Check sheet for the modelled part. Datum: model origin and axes. Units: mm. A direction names the side the tool comes from. Coordinates: 2 decimals unless noted, no trailing zeros. Loops run counter-clockwise (first coordinate to the right, second up) from the corner with the lowest first, then second, coordinate; pieces in that order, holes last. Notation, with made-up numbers: (-20, -24.75) -> (19, -24.75) arc R32 cw to (19, 7.25) -> close; hole circle Ø1 at (31, 58.25). An arc over 180 degrees is marked (long way). Use CSV: the item, a comma, the result in double quotes.
```python
from build123d import *

# Parameters (mm, degrees)
MODEL_R             = 2.5
MODEL_R_2           = 1.75
MODEL_W             = 40
MODEL_H             = 24
BOSS_EXTRUDE1_DEPTH = 12


with BuildPart() as part:
    # Model → Boss-Extrude1 (new body)
    with BuildSketch(Plane.XY):
        Polygon((5, 275), (0, 270), (0, 5), (5, 0), (125, 0), (130, 5), (130, 270), (125, 275), align=None)
        with Locations((16.49, 6.5)):
            Circle(MODEL_R, mode=Mode.SUBTRACT)
        with Locations((48.83, 6.5)):
            Circle(MODEL_R, mode=Mode.SUBTRACT)
        with Locations((81.17, 6.5)):
            Circle(MODEL_R, mode=Mode.SUBTRACT)
        with Locations((113.51, 6.5)):
            Circle(MODEL_R, mode=Mode.SUBTRACT)
        with Locations((29, 128.5)):
            Circle(MODEL_R_2, mode=Mode.SUBTRACT)
        with Locations((65, 128.5)):
            Circle(MODEL_R_2, mode=Mode.SUBTRACT)
        with Locations((101, 128.5)):
            Circle(MODEL_R_2, mode=Mode.SUBTRACT)
        with Locations((101, 93.5)):
            Circle(MODEL_R_2, mode=Mode.SUBTRACT)
        with Locations((65, 93.5)):
            Circle(MODEL_R_2, mode=Mode.SUBTRACT)
        with Locations((29, 93.5)):
            Circle(MODEL_R_2, mode=Mode.SUBTRACT)
        with Locations((29, 267.5)):
            Circle(MODEL_R_2, mode=Mode.SUBTRACT)
        with Locations((65, 267.5)):
            Circle(MODEL_R_2, mode=Mode.SUBTRACT)
        with Locations((101, 267.5)):
            Circle(MODEL_R_2, mode=Mode.SUBTRACT)
        with Locations((101, 232.5)):
            Circle(MODEL_R_2, mode=Mode.SUBTRACT)
        with Locations((65, 232.5)):
            Circle(MODEL_R_2, mode=Mode.SUBTRACT)
        with Locations((29, 232.5)):
            Circle(MODEL_R_2, mode=Mode.SUBTRACT)
        with Locations((15, 198.5)):
            Circle(MODEL_R_2, mode=Mode.SUBTRACT)
        with Locations((15, 173.5)):
            Circle(MODEL_R_2, mode=Mode.SUBTRACT)
        with Locations((15, 148.5)):
            Circle(MODEL_R_2, mode=Mode.SUBTRACT)
        with Locations((15, 123.5)):
            Circle(MODEL_R_2, mode=Mode.SUBTRACT)
        with Locations((15, 98.5)):
            Circle(MODEL_R_2, mode=Mode.SUBTRACT)
        with Locations((15, 73.5)):
            Circle(MODEL_R_2, mode=Mode.SUBTRACT)
        with Locations((15, 48.5)):
            Circle(MODEL_R_2, mode=Mode.SUBTRACT)
        with Locations((15, 23.5)):
            Circle(MODEL_R_2, mode=Mode.SUBTRACT)
        with Locations((115, 23.5)):
            Circle(MODEL_R_2, mode=Mode.SUBTRACT)
        with Locations((115, 48.5)):
            Circle(MODEL_R_2, mode=Mode.SUBTRACT)
        with Locations((115, 73.5)):
            Circle(MODEL_R_2, mode=Mode.SUBTRACT)
        with Locations((115, 98.5)):
            Circle(MODEL_R_2, mode=Mode.SUBTRACT)
        with Locations((115, 123.5)):
            Circle(MODEL_R_2, mode=Mode.SUBTRACT)
        with Locations((115, 148.5)):
            Circle(MODEL_R_2, mode=Mode.SUBTRACT)
        with Locations((115, 173.5)):
            Circle(MODEL_R_2, mode=Mode.SUBTRACT)
        with Locations((115, 198.5)):
            Circle(MODEL_R_2, mode=Mode.SUBTRACT)
        with Locations((65, 111)):
            Rectangle(MODEL_W, MODEL_H, mode=Mode.SUBTRACT)
        with BuildLine():
            Line((13.99, 163.82), (13.99, 160.82))
            ThreePointArc((13.99, 160.82), (16.49, 158.32), (18.99, 160.82))
            Line((18.99, 160.82), (18.99, 163.82))
            ThreePointArc((18.99, 163.82), (16.49, 166.32), (13.99, 163.82))
        make_face(mode=Mode.SUBTRACT)
        with BuildLine():
            Line((46.33, 163.82), (46.33, 160.82))
            ThreePointArc((46.33, 160.82), (48.83, 158.32), (51.33, 160.82))
            Line((51.33, 160.82), (51.33, 163.82))
            ThreePointArc((51.33, 163.82), (48.83, 166.32), (46.33, 163.82))
        make_face(mode=Mode.SUBTRACT)
        with BuildLine():
            Line((78.67, 163.82), (78.67, 160.82))
            ThreePointArc((78.67, 160.82), (81.17, 158.32), (83.67, 160.82))
            Line((83.67, 160.82), (83.67, 163.82))
            ThreePointArc((83.67, 163.82), (81.17, 166.32), (78.67, 163.82))
        make_face(mode=Mode.SUBTRACT)
        with BuildLine():
            Line((111.01, 163.82), (111.01, 160.82))
            ThreePointArc((111.01, 160.82), (113.51, 158.32), (116.01, 160.82))
            Line((116.01, 160.82), (116.01, 163.82))
            ThreePointArc((116.01, 163.82), (113.51, 166.32), (111.01, 163.82))
        make_face(mode=Mode.SUBTRACT)
        with BuildLine():
            Line((13.99, 217), (13.99, 214))
            ThreePointArc((13.99, 214), (16.49, 211.5), (18.99, 214))
            Line((18.99, 214), (18.99, 217))
            ThreePointArc((18.99, 217), (16.49, 219.5), (13.99, 217))
        make_face(mode=Mode.SUBTRACT)
        with BuildLine():
            Line((51.33, 214), (51.33, 217))
            ThreePointArc((51.33, 217), (48.83, 219.5), (46.33, 217))
            Line((46.33, 217), (46.33, 214))
            ThreePointArc((46.33, 214), (48.83, 211.5), (51.33, 214))
        make_face(mode=Mode.SUBTRACT)
        with BuildLine():
            Line((83.67, 214), (83.67, 217))
            ThreePointArc((83.67, 217), (81.17, 219.5), (78.67, 217))
            Line((78.67, 217), (78.67, 214))
            ThreePointArc((78.67, 214), (81.17, 211.5), (83.67, 214))
        make_face(mode=Mode.SUBTRACT)
        with BuildLine():
            Line((116.01, 214), (116.01, 217))
            ThreePointArc((116.01, 217), (113.51, 219.5), (111.01, 217))
            Line((111.01, 217), (111.01, 214))
            ThreePointArc((111.01, 214), (113.51, 211.5), (116.01, 214))
        make_face(mode=Mode.SUBTRACT)
        with BuildLine():
            Line((18.99, 58.18), (18.99, 61.18))
            ThreePointArc((18.99, 61.18), (16.49, 63.68), (13.99, 61.18))
            Line((13.99, 61.18), (13.99, 58.18))
            ThreePointArc((13.99, 58.18), (16.49, 55.68), (18.99, 58.18))
        make_face(mode=Mode.SUBTRACT)
        with BuildLine():
            Line((51.33, 58.18), (51.33, 61.18))
            ThreePointArc((51.33, 61.18), (48.83, 63.68), (46.33, 61.18))
            Line((46.33, 61.18), (46.33, 58.18))
            ThreePointArc((46.33, 58.18), (48.83, 55.68), (51.33, 58.18))
        make_face(mode=Mode.SUBTRACT)
        with BuildLine():
            Line((83.67, 58.18), (83.67, 61.18))
            ThreePointArc((83.67, 61.18), (81.17, 63.68), (78.67, 61.18))
            Line((78.67, 61.18), (78.67, 58.18))
            ThreePointArc((78.67, 58.18), (81.17, 55.68), (83.67, 58.18))
        make_face(mode=Mode.SUBTRACT)
        with BuildLine():
            Line((116.01, 58.18), (116.01, 61.18))
            ThreePointArc((116.01, 61.18), (113.51, 63.68), (111.01, 61.18))
            Line((111.01, 61.18), (111.01, 58.18))
            ThreePointArc((111.01, 58.18), (113.51, 55.68), (116.01, 58.18))
        make_face(mode=Mode.SUBTRACT)
        with Locations((65, 250)):
            Rectangle(MODEL_W, MODEL_H, mode=Mode.SUBTRACT)
    extrude(amount=BOSS_EXTRUDE1_DEPTH)


solid = part.part
```
1) Thickness scan on line 1 along X through (y, z) = (215.5, 4.5); line 2 along Y through (x, z) = (76.5, 8.5); line 3 along X through (y, z) = (148.5, 9.75). Record the ranges inside material, lowest first. Write a range as from..to.
Answer below:
line 1,"x = 0..13.99, 18.99..46.33, 51.33..78.67, 83.67..111.01, 116.01..130"
line 2,"y = 0..99, 123..238, 262..275"
line 3,"x = 0..13.25, 16.75..113.25, 116.75..130"
2) Cross-section at A-A on y = 115. Record the boundary of the cut face in (x, z), and give its area (3 significant figures).
Answer below:
outline,"(0, 0) -> (45, 0) -> (45, 12) -> (0, 12) -> close; (85, 0) -> (130, 0) -> (130, 12) -> (85, 12) -> close"
area,"1,080 mm²"
3) Cross-section at D-D on z = 2. Give the number of separate pieces and of enclosed holes in the cut face, and give its area (3 significant figures).
Answer below:
separate pieces,"1"
enclosed holes,"46"
area,"33,000 mm²"
4) Draft check along X on faces 1 (the flat face through (3, 273, 6)), 2 (the flat face through (66, 275, 6)), 3 (the cylindrical face through (16.54, 63.68, 5.92)). Enter one of: released by +X, released by -X, zero draft, split by the parting line, or undercut.
Answer below:
face 1,"released by -X"
face 2,"zero draft"
face 3,"undercut"
5) Cross-section at B-B on x = 81.17. Record the boundary of the cut face in (y, z), and give its area (3 significant figures).
Answer below:
outline,"(0, 0) -> (4, 0) -> (4, 12) -> (0, 12) -> close; (9, 0) -> (55.68, 0) -> (55.68, 12) -> (9, 12) -> close; (63.68, 0) -> (99, 0) -> (99, 12) -> (63.68, 12) -> close; (123, 0) -> (158.32, 0) -> (158.32, 12) -> (123, 12) -> close; (166.32, 0) -> (211.5, 0) -> (211.5, 12) -> (166.32, 12) -> close; (219.5, 0) -> (238, 0) -> (238, 12) -> (219.5, 12) -> close; (262, 0) -> (275, 0) -> (275, 12) -> (262, 12) -> close"
area,"2,380 mm²"
6) Go/stop test with a flat-tipped pin: pin 1 Ø1.5 at (y, z) = (161.5, 3.5) entering from -X. Record where the tip stops, or that it passes through.
Answer below:
pin 1,"stops at x = 0"
7) Cross-section at C-C on x = 59. Record the boundary of the cut face in (y, z).
Answer below:
outline,"(0, 0) -> (99, 0) -> (99, 12) -> (0, 12) -> close; (123, 0) -> (238, 0) -> (238, 12) -> (123, 12) -> close; (262, 0) -> (275, 0) -> (275, 12) -> (262, 12) -> close"
8) Access from +Z, -Z, +X, -X, +Y, -Y to the whole of each face (thin tool, end or side, straight path). Record for faces 4 (the flat face through (64, 139, 12)), 5 (the cylindrical face through (48.88, 166.32, 5.92)).
Answer below:
face 4,"+Z, +X, -X, +Y, -Y"
face 5,"+Z, -Z"
